Work out the finished part from the listing and answer in its coordinate system (mm). A direction names the side the tool comes from. Coordinates: 2 decimals unless noted, no trailing zeros. Loops run counter-clockwise (first coordinate to the right, second up) from the corner with the lowest first, then second, coordinate; pieces in that order, holes last. Notation, with made-up numbers: (88.25, -1.5) - (106.25, -1.5) arc R12 cw to (106.25, 11.5) - close; hole circle Ø3 at (60, 62.5). An arc over 180 degrees is marked (long way). Write each question's results on one line, items separated by ' | '. Start each with the question number.
Item 1: Section C-C, the plane x = -3 is taken. Write down the section's boundary in (y, z), plus the area to 3 significant figures.
Item 2: This flat-tipped pin is pushed along its axis until it touches: pin 1 Ø19 at (x, y) = (59, -3.5) entering from -Z. Where does it stop, or does it pass through?
Item 3: Section B-B, the plane z = 24 is taken. Write down the section's boundary in (x, y), plus the area to 3 significant figures.
Item 4: Consider probe 1 along Y at (x, z) = (59, 34); probe 2 along Z at (x, y) = (90.5, 5). Determine where each line is inside the solid, lowest interval first. Write a range as [from, to].
Item 5: For a pull along Z with two mould halves and no side action, classify faces 3 (the face through (30.95, -3.58, 49.65)), 4 (the face through (60, 13, 0)), 5 (the face through (60, -19.667, 25)), 6 (the face through (60, 12, 0.683)) as +Z half, -Z half, draft (parallel to the pull), parting line (faces both ways), or undercut.
Item 6: A tool of negligible diameter and unlimited length cuts with its end or side. For faces 1 (the face through (60, 12, 49.317)), 2 (the face through (33.37, 31.78, 0.34)), from which of +Z, -Z, +X, -X, +Y, -Y can it reach the whole face along a straight path? Write none if from no direction.
Item 7: Section A-A, the plane y = 36.5 is taken. Write down the section's boundary in (x, z), plus the area to 3 significant figures.
from build123d import *

# Parameters (mm, degrees)
ESBO_O1_W                = 150
ESBO_O1_H                = 50
ESBO_O1_R                = 1.35
RESSALTO_EXTRUS_O1_DEPTH = 50
ESBO_O5_W                = 150
ESBO_O5_H                = 14.978385154
RESSALTO_EXTRUS_O2_DEPTH = 50
ESBO_O6_W                = 48.634106334
ESBO_O6_H                = 63.528836918
CORTE_EXTRUS_O6_DEPTH    = 165.280193846


with BuildPart() as part:
    # Esboço1 → Ressalto-extrusão1 (new body)
    with BuildSketch(Plane.XY):
        with Locations((61.085582475, 19.586792778)):
            Rectangle(ESBO_O1_W, ESBO_O1_H)
        with Locations((-11.702376595, -3.638707723)):
            Circle(ESBO_O1_R, mode=Mode.SUBTRACT)
        with Locations((10.297623405, -3.638707723)):
            Circle(ESBO_O1_R, mode=Mode.SUBTRACT)
        with Locations((32.297623405, -3.638707723)):
            Circle(ESBO_O1_R, mode=Mode.SUBTRACT)
        with Locations(Location((32.297623405, 30.961292277, 0), (0, 0, 180))):
            Circle(ESBO_O1_R, mode=Mode.SUBTRACT)
        with Locations(Location((10.297623405, 30.961292277, 0), (0, 0, 180))):
            Circle(ESBO_O1_R, mode=Mode.SUBTRACT)
        with Locations(Location((-11.702376595, 30.961292277, 0), (0, 0, 180))):
            Circle(ESBO_O1_R, mode=Mode.SUBTRACT)
    extrude(amount=RESSALTO_EXTRUS_O1_DEPTH)

    # Esboço5 → Ressalto-extrusão2 (add)
    with BuildSketch(Plane.XY.offset(50)):
        with Locations((61.085582475, -12.902399799)):
            Rectangle(ESBO_O5_W, ESBO_O5_H)
    extrude(amount=-RESSALTO_EXTRUS_O2_DEPTH)

    # Esboço6 → Corte-extrusão6 (cut, through all)
    with BuildSketch(Plane.ZY.offset(13.914417525)):
        with Locations((25, 12.097600201)):
            Rectangle(ESBO_O6_W, ESBO_O6_H)
    extrude(amount=-CORTE_EXTRUS_O6_DEPTH, mode=Mode.SUBTRACT)


solid = part.part
Answer key:
1) outline: (-20.39, 0) - (44.59, 0) - (44.59, 50) - (-20.39, 50) - close; hole (-19.67, 0.68) - (43.86, 0.68) - (43.86, 49.32) - (-19.67, 49.32) - close | area: 159 mm^2
2) pin 1: stops at z = 0
3) outline: (-13.91, -20.39) - (136.09, -20.39) - (136.09, -19.67) - (-13.91, -19.67) - close; (-13.91, 43.86) - (136.09, 43.86) - (136.09, 44.59) - (-13.91, 44.59) - close | area: 217 mm^2
4) probe 1: y = [-20.39, -19.67], [43.86, 44.59] | probe 2: z = [0, 0.68], [49.32, 50]
5) face 3: draft | face 4: -Z half | face 5: undercut | face 6: undercut
6) face 1: +X, -X | face 2: +Z, -Z
7) outline: (-13.91, 0) - (136.09, 0) - (136.09, 0.68) - (-13.91, 0.68) - close; (-13.91, 49.32) - (136.09, 49.32) - (136.09, 50) - (-13.91, 50) - close | area: 205 mm^2
